```python
from build123d import *

# Parameters (mm, degrees)
BOSS_EXTRU_1_DEPTH      = 8
ENL_V_MAT_EXTRU_1_DEPTH = 8


with BuildPart() as part:
    # Esquisse1 → Boss.-Extru.1 (new body)
    with BuildSketch(Plane.XY):
        with BuildLine():
            Line((30.121320344, 221.336361724), (36, 221.336361724))
            Line((36, 221.336361724), (36, 171.336361724))
            Line((36, 171.336361724), (30.121320344, 171.336361724))
            ThreePointArc((30.121320344, 171.336361724), (28.201672528, 171.196524964), (28, 169.282385406))
            Line((28, 169.282385406), (28, 151.336361724))
            Line((28, 151.336361724), (-242, 151.336361724))
            Line((-242, 151.336361724), (-242, 171.40370575))
            Line((-242, 171.40370575), (-236.121320344, 171.40370575))
            ThreePointArc((-236.121320344, 171.40370575), (-234, 171.40370575), (-234, 173.525026093))
            Line((-234, 173.525026093), (-234, 219.282385406))
            ThreePointArc((-234, 219.282385406), (-234.201672528, 221.196524964), (-236.121320344, 221.336361724))
            Line((-236.121320344, 221.336361724), (-242, 221.336361724))
            Line((-242, 221.336361724), (-242, 241.336361724))
            Line((-242, 241.336361724), (-224.049400042, 241.336361724))
            ThreePointArc((-224.049400042, 241.336361724), (-221.965737315, 241.439112813), (-222, 243.525026093))
            Line((-222, 243.525026093), (-222, 249.336361724))
            Line((-222, 249.336361724), (-172, 249.336361724))
            Line((-172, 249.336361724), (-172, 243.525026093))
            ThreePointArc((-172, 243.525026093), (-172.034262685, 241.439112813), (-169.950599958, 241.336361724))
            Line((-169.950599958, 241.336361724), (-44.121320344, 241.336361724))
            ThreePointArc((-44.121320344, 241.336361724), (-42, 241.336361724), (-42, 243.457682068))
            Line((-42, 243.457682068), (-42, 249.336361724))
            Line((-42, 249.336361724), (8, 249.336361724))
            Line((8, 249.336361724), (8, 243.457682068))
            ThreePointArc((8, 243.457682068), (8, 241.336361724), (10.121320344, 241.336361724))
            Line((10.121320344, 241.336361724), (28, 241.336361724))
            Line((28, 241.336361724), (28, 223.525026093))
            ThreePointArc((28, 223.525026093), (27.966327987, 221.370033737), (30.121320344, 221.336361724))
        make_face()
    extrude(amount=BOSS_EXTRU_1_DEPTH)

    # Esquisse2 → Enlèv. mat.-Extru.1 (cut)
    with BuildSketch(Plane.XY.offset(8)):
        with BuildLine():
            Line((3.5, 221.336361724), (3.5, 171.336361724))
            ThreePointArc((3.5, 171.336361724), (-4, 163.836361724), (-11.5, 171.336361724))
            Line((-11.5, 171.336361724), (-11.5, 221.336361724))
            ThreePointArc((-11.5, 221.336361724), (-4, 228.836361724), (3.5, 221.336361724))
        make_face()
        with BuildLine():
            Line((-196.761984324, 211.248045222), (-196.738010886, 181.248045222))
            ThreePointArc((-196.738010886, 181.248045222), (-189.232019924, 173.754040975), (-181.738015676, 181.260031937))
            Line((-181.738015676, 181.260031937), (-181.761989114, 211.260031937))
            ThreePointArc((-181.761989114, 211.260031937), (-189.267980076, 218.754036185), (-196.761984324, 211.248045222))
        make_face()
    extrude(amount=-ENL_V_MAT_EXTRU_1_DEPTH, mode=Mode.SUBTRACT)


solid = part.part
```
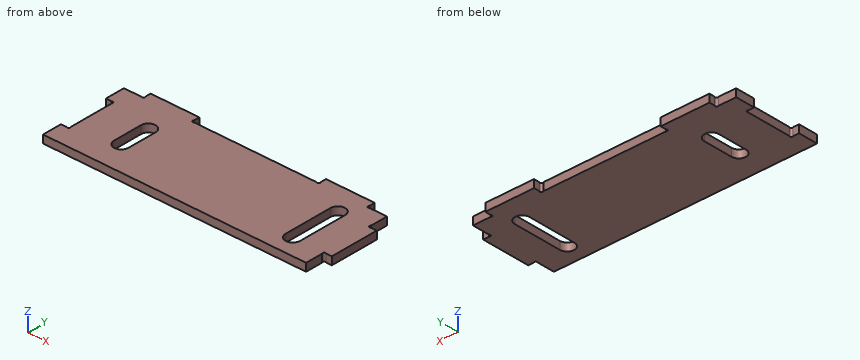
Model file for the job. Use its own axes, mm. Coordinates: 2 decimals unless noted, no trailing zeros. Loops run counter-clockwise (first coordinate to the right, second up) from the corner with the lowest first, then second, coordinate; pieces in that order, holes last. Notation, with made-up numbers: (89.5, -8) -> (102.5, -8) arc R22 cw to (102.5, 31) -> close; hole circle Ø6 at (6, 64). An arc over 180 degrees is marked (long way). Answer as a JSON object with one key per item and string values.
Q1. Cut at C-C (y = 215). List the corners of the cut face in (x, z).
Report:
{"outline": "(-234, 0) -> (-195.76, 0) -> (-195.76, 8) -> (-234, 8) -> close; (-182.76, 0) -> (-11.5, 0) -> (-11.5, 8) -> (-182.76, 8) -> close; (3.5, 0) -> (36, 0) -> (36, 8) -> (3.5, 8) -> close"}
Q2. Cut at B-B (z = 5.75). State how many separate pieces and enclosed holes the cut face has, and give its area (3 significant figures).
Report:
{"separate pieces": "1", "enclosed holes": "2", "area": "23,500 mm2"}
Q3. Flat gauge pins, fed straight in: P1, Ø1.8, axis at y = 245.5, z = 3, coming from the -X side; P2, Ø2.5, axis at x = 21, z = 5, coming from the +Y side; P3, Ø4.5, axis at x = 33, z = 5, coming from the +Y side; P4, Ø1, axis at x = -26.5, y = 233.5, coming from the -Z side. Where does each tip first touch, or does it go through?
Report:
{"P1": "stops at x = -222", "P2": "stops at y = 241.34", "P3": "stops at y = 221.34", "P4": "stops at z = 0"}
Q4. Cut at A-A (x = -4). List the corners of the cut face in (y, z).
Report:
{"outline": "(151.34, 0) -> (163.84, 0) -> (163.84, 8) -> (151.34, 8) -> close; (228.84, 0) -> (249.34, 0) -> (249.34, 8) -> (228.84, 8) -> close"}
Q5. Probe probe 1 along X at (y, z) = (190, 4.25) (3 decimals); probe 2 along X at (y, z) = (245.5, 7.75); probe 3 along X at (y, z) = (210, 6.75). List the from-to ranges inside material, lowest first.
Report:
{"probe 1": "x = -234 to -196.745, -181.745 to -11.5, 3.5 to 36", "probe 2": "x = -222 to -172, -42 to 8", "probe 3": "x = -234 to -196.76, -181.76 to -11.5, 3.5 to 36"}
Q6. Cut at D-D (x = -191). List the corners of the cut face in (y, z).
Report:
{"outline": "(151.34, 0) -> (173.96, 0) -> (173.96, 8) -> (151.34, 8) -> close; (218.55, 0) -> (249.34, 0) -> (249.34, 8) -> (218.55, 8) -> close"}
